from build123d import *

# Parameters (mm, degrees)
SKETCH1_R           = 13.8327
SKETCH1_R_2         = 13.15
BOSS_EXTRUDE1_DEPTH = 3
BOSS_EXTRUDE2_START = 1
SKETCH2_R           = 13.8327
SKETCH2_R_2         = 9.525
BOSS_EXTRUDE2_DEPTH = 1
BOSS_EXTRUDE3_START = 3
SKETCH3_R           = 13.8327
SKETCH3_R_2         = 13.15
BOSS_EXTRUDE3_DEPTH = 3
FILLET1_R           = 0.5


with BuildPart() as part:
    # Sketch1 → Boss-Extrude1 (new body)
    with BuildSketch(Plane.XY):
        Circle(SKETCH1_R)
        Circle(SKETCH1_R_2, mode=Mode.SUBTRACT)
    extrude(amount=-BOSS_EXTRUDE1_DEPTH)

    # Sketch2 → Boss-Extrude2 (add)
    with BuildSketch(Plane.XY.offset(BOSS_EXTRUDE2_START)):
        Circle(SKETCH2_R)
        Circle(SKETCH2_R_2, mode=Mode.SUBTRACT)
    extrude(amount=-BOSS_EXTRUDE2_DEPTH)

    # Sketch3 → Boss-Extrude3 (add)
    with BuildSketch(Plane.XY.offset(1).offset(BOSS_EXTRUDE3_START)):
        Circle(SKETCH3_R)
        Circle(SKETCH3_R_2, mode=Mode.SUBTRACT)
    extrude(amount=-BOSS_EXTRUDE3_DEPTH)

    # Fillet1
    fillet1_edges = [part.edges().sort_by_distance(p)[0] for p in [
        (-13.15, 0, 0),
        (-13.15, 0, 1),
    ]]
    fillet(fillet1_edges, radius=FILLET1_R)


solid = part.part
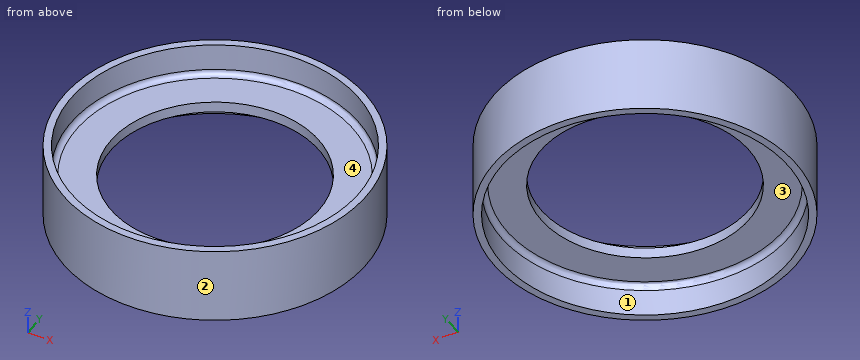
Could you check a few things on this model? Use its own coordinates, in mm. Face numbers are marked on the shaded views. A direction names the side the tool comes from. Give positions to 0.01 mm unless a question says otherwise; leave off trailing zeros. Order: outer loops, then holes, each group sorted by start corner. A loop starts at its lowest first (then second) coordinate and runs counter-clockwise, first axis right, second up. Notation, with made-up numbers: (88, 41.25) - (124, 41.25) arc R12 cw to (124, 51.25) - close; hole circle Ø2 at (88.5, 14.25). An arc over 180 degrees is marked (long way). One line per question, with ' | ' between items. Start each with the question number.
Item 1: I'm going to push flat-ended pins straight in: pin 1 Ø2 at (y, z) = (-9, -0.5) entering from -X; pin 2 Ø1 at (x, z) = (7.5, -1.5) entering from +Y; pin 3 Ø12.5 at (x, y) = (-5, -4.5) entering from -Z; pin 4 Ø5 at (x, y) = (-10.5, -4) entering from +Z. Where does each tip first touch, or does it pass through?
Item 2: I want a section at A-A on x = 0. Write out the boundary of the cut face in (y, z) (3 decimals), then the cut area to 3 significant figures.
Item 3: I want a section at C-C on z = 3.5. Write out the boundary of the cut face in (x, y), then the cut area to 3 significant figures.
Item 4: I need wall thicknesses on probe 1 along Y at (x, z) = (0, 0.75) (3 decimals); probe 2 along Z at (x, y) = (11.5, -2.25); probe 3 along Y at (x, z) = (9.75, -0.25). Which ranges of each line are inside material? Lowest first, please. Write a range as [from, to].
Item 5: For the marked faces 3 and 4, which set-ups out of +Z, -Z, +X, -X, +Y, -Y let a thin tool reach every point of the face, with its end or its side?
Item 6: I want a section at D-D on z = 0.5. Write out the boundary of the cut face in (x, y) (3 decimals).
Item 7: Thinking about a two-plate mould opening in Y: for the marked faces 1 and 2, which applies, pulls with the +Y half, pulls with the -Y half, needs draft (parallel to the pull), parting line crosses it, or undercut?
Verdict:
1) pin 1: x = -11.28 | pin 2: y = 11.93 | pin 3: z = -0.12 | pin 4: z = 4
2) outline: (-13.833, -3) - (-13.15, -3) - (-13.15, -0.5) arc R0.5 cw to (-12.65, 0) - (-9.525, 0) - (-9.525, 1) - (-12.65, 1) arc R0.5 cw to (-13.15, 1.5) - (-13.15, 4) - (-13.833, 4) - close; (9.525, 0) - (12.65, 0) arc R0.5 cw to (13.15, -0.5) - (13.15, -3) - (13.833, -3) - (13.833, 4) - (13.15, 4) - (13.15, 1.5) arc R0.5 cw to (12.65, 1) - (9.525, 1) - close | area: 17.0 mm^2
3) outline: circle Ø27.67 at (0, 0); hole circle Ø26.3 at (0, 0) | area: 57.9 mm^2
4) probe 1: [-13.833, -9.525], [9.525, 13.833] | probe 2: [0, 1] | probe 3: [-9.81, -8.72], [8.72, 9.81]
5) face 3: -Z | face 4: +Z
6) outline: circle Ø27.665 at (0, 0); hole circle Ø19.05 at (0, 0)
7) face 1: undercut | face 2: parting line crosses it
